Job drawing, mm, ordinate dimensions from the low corner. One solid piece. Round coordinates to 2 decimals unless told otherwise and drop trailing zeros. Write each loop counter-clockwise with the first axis right and the second up, starting at its lowest first coordinate (ties: lowest second). Pieces come first, ordered by that corner, then holes. Notation, with made-up numbers: (73.25, 1) - (99.25, 1) arc R19 ccw to (99.25, 15) - close; hole circle Ø7 at (25.25, -3). An arc over 180 degrees is marked (long way). Write each question's results on one line, items separated by ' | '.
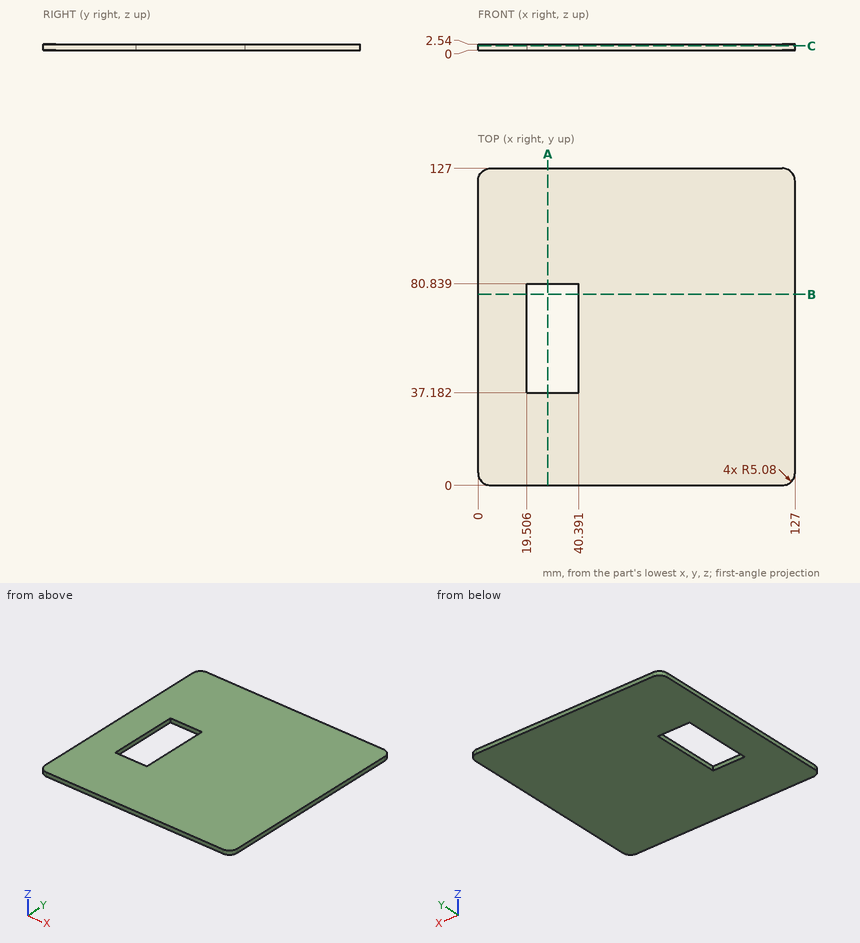
(1) Drill centre lines: probe 1 along X at (y, z) = (42, 0.6); probe 2 along Y at (x, z) = (39, 1.75); probe 3 along Y at (x, z) = (122, 1.25). Where is each one in solid material? Low to high. Write a range as [from, to].
Worked answers:
probe 1: x = [0, 19.51], [40.39, 127] | probe 2: y = [0, 37.18], [80.84, 127] | probe 3: y = [0, 127]
(2) Slice it at C-C, the plane z = 1.8. Write the cut outline in (x, y), and give its area (3 significant figures).
Worked answers:
outline: (0, 5.08) arc R5.08 ccw to (5.08, 0) - (121.92, 0) arc R5.08 ccw to (127, 5.08) - (127, 121.92) arc R5.08 ccw to (121.92, 127) - (5.08, 127) arc R5.08 ccw to (0, 121.92) - close; hole (19.51, 37.18) - (40.39, 37.18) - (40.39, 80.84) - (19.51, 80.84) - close | area: 15,200 mm2
(3) Slice it at B-B, the plane y = 76.5. Write the cut outline in (x, z).
Worked answers:
outline: (0, 0) - (19.51, 0) - (19.51, 2.54) - (0, 2.54) - close; (40.39, 0) - (127, 0) - (127, 2.54) - (40.39, 2.54) - close
(4) Slice it at A-A, the plane x = 28. Write the cut outline in (y, z).
Worked answers:
outline: (0, 0) - (37.18, 0) - (37.18, 2.54) - (0, 2.54) - close; (80.84, 0) - (127, 0) - (127, 2.54) - (80.84, 2.54) - close
